Model file for the job. Use its own axes, mm. Round coordinates to 2 decimals unless told otherwise and drop trailing zeros. Order: outer loops, then holes, each group sorted by start corner. A loop starts at its lowest first (then second) coordinate and runs counter-clockwise, first axis right, second up. Notation, with made-up numbers: (69, -35.5) -> (106, -35.5) arc R19 ccw to (106, -15.5) -> close; hole circle Ø1 at (-10.75, 2). An arc over 180 degrees is marked (long way). Answer as CSV lines item,"result".
Autodesk Inventor part; units mm, degrees
ref_plane "YZ Plane" through (0, 0, 0) normal (1, 0, 0) x (0, 1, 0)
ref_plane "XZ Plane" through (0, 0, 0) normal (0, 1, 0) x (-1, 0, 0)
ref_plane "XY Plane" through (0, 0, 0) normal (0, 0, 1) x (1, 0, 0)
sketch "Sketch1" plane through (0, 0, 0) normal (0, 1, 0) x (-1, 0, 0)
  line L0 (-245, 255) -> (245, 255)
  line L1 (245, 255) -> (245, -255)
  line L2 (245, -255) -> (-245, -255)
  line L3 (-245, -255) -> (-245, 255)
  line L4 (-245, 255) -> (245, -255) construction
  line L5 (245, 255) -> (-245, -255) construction
  line L6 (225, 255) -> (225, 235)
  line L7 (225, 235) -> (245, 235)
  line L8 (225, -255) -> (225, -235)
  line L9 (225, -235) -> (245, -235)
  line L10 (-225, 255) -> (-225, 235)
  line L11 (-225, 235) -> (-245, 235)
  line L12 (-225, -255) -> (-225, -235)
  line L13 (-225, -235) -> (-245, -235)
  point P0 (0, 0)
  dimension "d0" = 510
  dimension "d1" = 490
  dimension "d2" = 20
extrude "Extrusion2" add sketch "Sketch1" along normal mid plane 3 contours L0 L6 L7 L1 L9 L8 L2 L12 L13 L3 L11 L10
sketch "Sketch2" plane through (0, -1.5, 0) normal (0, -1, 0) x (1, 0, 0)
  line L0 (235, -245) -> (-235, -245) construction
  line L1 (-235, -245) -> (-235, 245) construction
  line L2 (-235, 245) -> (235, 245) construction
  line L3 (235, 245) -> (235, -245) construction
  line L4 (235, -245) -> (-235, 245) construction
  line L5 (-235, -245) -> (235, 245) construction
  line L6 (-245, 235) -> (-245, -235) construction
  line L7 (225, 255) -> (-225, 255) construction
  circle A0 centre (-235, 98) radius 2.1
  circle A1 centre (-235, -98) radius 2.1
  circle A2 centre (-110, -245) radius 2.1
  circle A3 centre (110, -245) radius 2.1
  circle A4 centre (235, -127.5) radius 2.1
  circle A5 centre (235, 127.5) radius 2.1
  circle A6 centre (135, 245) radius 2.1
  circle A7 centre (-110, 245) radius 2.1
  line L8 (-245, 0) -> (245, 0) construction
  line L9 (-225, 255) -> (225, 255) construction
  line L10 (0, 255) -> (0, -257) construction
  point P0 (0, 0)
  point P1 (0, 0)
  point P2 (0, 0)
  dimension "d7" = 10
  dimension "d8" = 10
  dimension "d9" = 117.5
  dimension "d10" = 100
  dimension "d11" = 4.2
  dimension "d27" = 147
extrude "Extrusion3" cut sketch "Sketch2" against normal through all
sketch "Sketch3" plane through (0, -1.5, 0) normal (0, -1, 0) x (1, 0, 0)
  line L0 (-205, -15.5) -> (-174, -15.5) construction
  line L1 (-174, -15.5) -> (-174, 15.5) construction
  line L2 (-174, 15.5) -> (-205, 15.5) construction
  line L3 (-205, 15.5) -> (-205, -15.5) construction
  line L4 (-205, -15.5) -> (-174, 15.5) construction
  line L5 (-174, -15.5) -> (-205, 15.5) construction
  line L6 (-245, 235) -> (-245, -235)
  line L7 (0, 0) -> (-245, 0) construction
  circle A0 centre (-189.5, 0) radius 11
  circle A1 centre (-205, 15.5) radius 1.7
  circle A2 centre (-174, 15.5) radius 1.7
  circle A3 centre (-174, -15.5) radius 1.7
  circle A4 centre (-205, -15.5) radius 1.7
  point P0 (-189.5, 0)
  dimension "d14" = 40
  dimension "d15" = 22
  dimension "d16" = 31
  dimension "d17" = 3.4
extrude "Extrusion4" cut sketch "Sketch3" against normal through all
sketch "Sketch4" plane through (0, -1.5, 0) normal (0, -1, 0) x (1, 0, 0)
  line L0 (-245, 111.25) -> (-225, 111.25)
  line L1 (-225, 111.25) -> (-225, 181.75)
  line L2 (-225, 181.75) -> (-245, 181.75)
  line L3 (-245, 181.75) -> (-245, 111.25)
  line L4 (-225, 235) -> (-245, 235)
  line L5 (-245, 235) -> (-245, -235)
  line L6 (-245, 146.5) -> (-216, 146.5) construction
  line L7 (-225, 140.25) -> (-216.5, 140.25)
  line L8 (-216.5, 140.25) -> (-216.5, 152.75)
  line L9 (-216.5, 152.75) -> (-225, 152.75)
  line L10 (-225, 152.75) -> (-225, 140.25)
  point P0 (0, 0)
  dimension "d21" = 70.5
  dimension "d22" = 12.5
  dimension "d23" = 8.5
  dimension "d28" = 20
  dimension "d29" = 88.5
extrude "Extrusion5" cut sketch "Sketch4" against normal through all
mirror "Mirror1" about plane through (0, 0, 0) normal (0, 0, 1) of "Extrusion5"
fillet "Fillet1" radius 1 12 edges at (-225, 0, -111.25) (-216.5, 0, -140.25) (-216.5, 0, -152.75) (-225, 0, -181.75) (-225, 0, -152.75) (-225, 0, -140.25) (-225, 0, 152.75) (-225, 0, 140.25) (-216.5, 0, 152.75) (-225, 0, 181.75) (-216.5, 0, 140.25) (-225, 0, 111.25)
sketch "Sketch6" plane through (0, -1.5, 0) normal (0, -1, 0) x (1, 0, 0)
  line L0 (-105, 185) -> (45, 185) construction
  line L1 (45, 185) -> (45, 135) construction
  line L2 (45, 135) -> (-105, 135) construction
  line L3 (-105, 135) -> (-105, 185) construction
  circle A0 centre (45, 185) radius 2.1
  circle A1 centre (45, 135) radius 2.1
  circle A2 centre (-105, 135) radius 2.1
  circle A3 centre (-105, 185) radius 2.1
  line L4 (225, 255) -> (-225, 255)
  line L5 (-245, 235) -> (-245, 181.75)
  point P0 (0, 0)
  dimension "d30" = 50
  dimension "d31" = 150
  dimension "d32" = 4.2
  dimension "d33" = 70
  dimension "d34" = 140
hole "Hole1" at (45, -1.5, 185) at (45, -1.5, 135) at (-105, -1.5, 135) at (-105, -1.5, 185) direction (0, 1, 0) diameter 4.2 end through all
sketch "Sketch7" plane through (0, -1.5, 0) normal (0, -1, 0) x (1, 0, 0)
  circle A0 centre (-205, 215) radius 10
  circle A1 centre (-205, -215) radius 10
  line L0 (-205, 215) -> (-205, -215) construction
  line L1 (0, 0) -> (-205, 0) construction
  line L2 (225, 255) -> (-225, 255) construction
  line L3 (-225, -112.25) -> (-225, -139.25) construction
  dimension "d50" = 20
  dimension "d51" = 40
  dimension "d52" = 20
extrude "Cut1" cut sketch "Sketch7" against normal blind 3
sketch "Sketch8" plane through (0, -1.5, 0) normal (0, -1, 0) x (1, 0, 0)
  line L0 (-20, 55) -> (-20, -7) construction
  line L1 (-20, -7) -> (-70, -7) construction
  line L2 (-70, -7) -> (-70, 55) construction
  line L3 (-70, 55) -> (-20, 55) construction
  line L4 (-70, 55) -> (-70, -7) construction
  line L5 (-70, -7) -> (-120, -7) construction
  line L6 (-120, -7) -> (-120, 55) construction
  line L7 (-120, 55) -> (-70, 55) construction
  line L8 (-45, 55) -> (-45, -2.575) construction
  line L9 (-95, 55) -> (-95, -7) construction
  line L10 (225, 255) -> (-225, 255) construction
  circle A0 centre (-45, 47.38) radius 2.1
  line L11 (-45, 1.85) -> (-45, -7) construction
  line L12 (-47.1, 1.85) -> (-47.1, -3.15)
  line L13 (-42.9, -3.15) -> (-42.9, 1.85)
  arc A1 (-42.9, 1.85) -> (-47.1, 1.85) centre (-45, 1.85) ccw
  arc A2 (-47.1, -3.15) -> (-42.9, -3.15) centre (-45, -3.15) ccw
  line L14 (-20, 24) -> (-120, 24) construction
  circle A3 centre (-95, 47.38) radius 2.1
  line L15 (-95, 1.85) -> (-95, -3.15) construction
  line L16 (-97.1, 1.85) -> (-97.1, -3.15)
  line L17 (-92.9, -3.15) -> (-92.9, 1.85)
  arc A4 (-92.9, 1.85) -> (-97.1, 1.85) centre (-95, 1.85) ccw
  arc A5 (-97.1, -3.15) -> (-92.9, -3.15) centre (-95, -3.15) ccw
  line L18 (-245, 111.25) -> (-245, -111.25)
  point P0 (0, 0)
  point P1 (-95, -0.65)
  point P2 (-70, 24)
  dimension "d56" = 50
  dimension "d57" = 62
  dimension "d58" = 45.53
  dimension "d59" = 7.62
  dimension "d60" = 5
  dimension "d61" = 4.2
  dimension "d66" = 200
  dimension "d67" = 175
extrude "Cut2" cut sketch "Sketch8" against normal blind 3
sketch "Sketch9" plane through (0, -1.5, 0) normal (0, -1, 0) x (1, 0, 0)
  line L0 (-119.2, -73.2) -> (-195, -73.2) construction
  line L1 (-195, -73.2) -> (-195, -175) construction
  line L2 (-195, -175) -> (-119.2, -175) construction
  line L3 (-119.2, -175) -> (-119.2, -73.2) construction
  line L4 (245, -235) -> (245, 235) construction
  circle A0 centre (-119.2, -73.2) radius 1.7
  circle A1 centre (-119.2, -175) radius 1.7
  circle A2 centre (-195, -175) radius 1.7
  circle A3 centre (-195, -73.2) radius 1.7
  line L5 (-225, -255) -> (225, -255)
  line L6 (-245, 111.25) -> (-245, -111.25)
  point P0 (0, 0)
  dimension "d68" = 101.8
  dimension "d69" = 75.8
  dimension "d71" = 3.4
  dimension "d74" = 80
  dimension "d75" = 50
extrude "Cut3" cut sketch "Sketch9" against normal blind 3
equation "\"d40\" = Thickness"
equation "\"d54\" = Thickness"
equation "\"d63\" = Thickness"
equation "\"d72\" = Thickness"
equation "\"CornerReliefSize\" = 4 * Thickness"
equation "\"TransitionRadius\" = BendRadius"
equation "\"JacobiRadiusSize\" = BendRadius"
equation "\"d53\" = Thickness"
properties part number "Internal Base Cladding" material "Aluminium 1050"
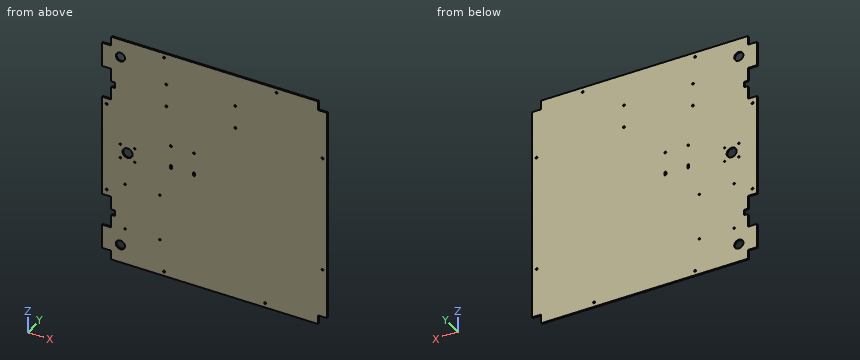
Q1. Flat gauge pins, fed straight in: pin 1 (0.9 mm diameter, centred on y = 0, z = 146, fed in from -X); pin 2 (5.5 mm diameter, centred on x = -105, z = 135, fed in from -Y); pin 3 (0.9 mm diameter, centred on y = 0, z = -129.5, fed in from -X). Where does each tip first touch, or does it go through?
Checks:
pin 1,"x = -216.5"
pin 2,"y = -1.5"
pin 3,"x = -225"
Q2. Saw through at A-A (z = -215). Write the cut outline in (x, y).
Checks:
outline,"(-245, -1.5) -> (-215, -1.5) -> (-215, 1.5) -> (-245, 1.5) -> close; (-195, -1.5) -> (245, -1.5) -> (245, 1.5) -> (-195, 1.5) -> close"
Q3. Saw through at B-B (y = -0.5). State how many separate pieces and enclosed holes the cut face has, plus the area to 3 significant figures.
Checks:
separate pieces,"1"
enclosed holes,"27"
area,"244,000 mm²"
Q4. Wall check: L1, parallel to X at y = -0.75, z = 185; L2, parallel to Z at x = -105, y = -0.7; L3, parallel to Z at x = -110, y = 0.6. Give the ranges that are in metal, low to high. Write a range as [from, to].
Checks:
L1,"[-245, -107.1], [-102.9, 42.9], [47.1, 245]"
L2,"[-255, 132.9], [137.1, 182.9], [187.1, 255]"
L3,"[-255, -247.1], [-242.9, 242.9], [247.1, 255]"
